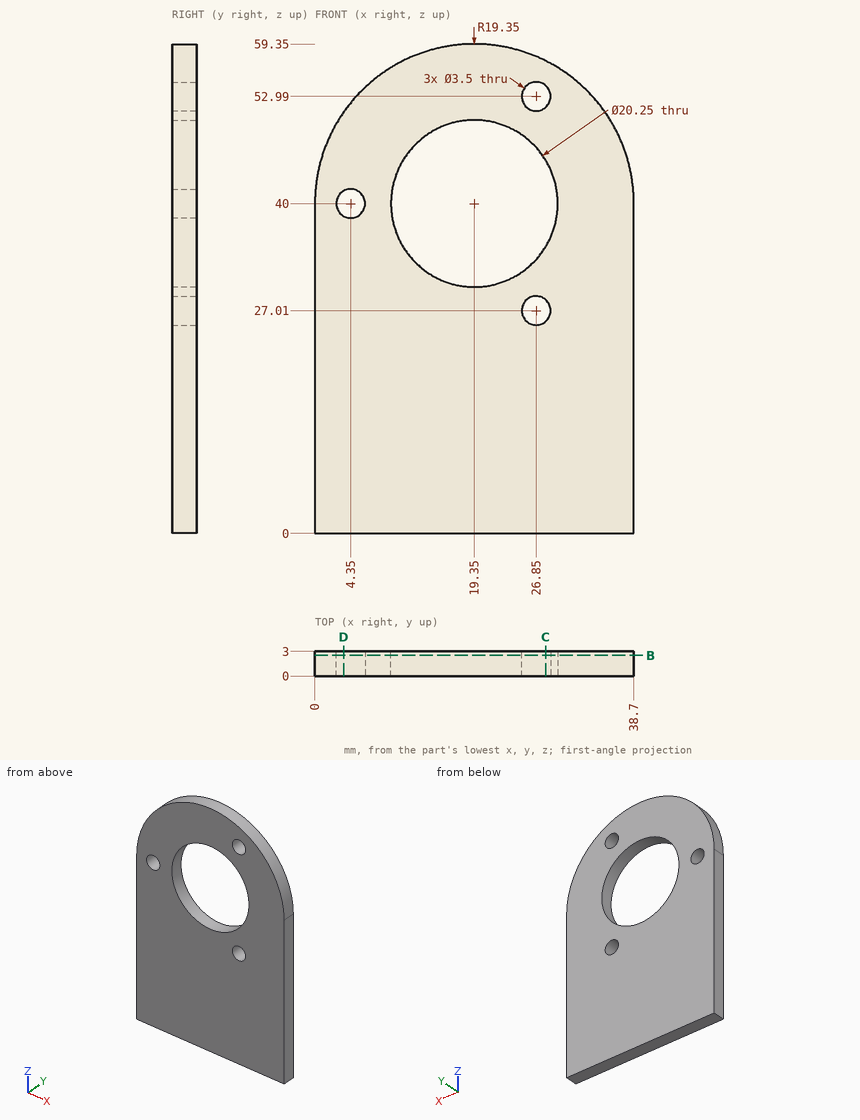
Drawing for the job (mm, zero at the part's lowest x, y, z). Give positions to 0.01 mm unless a question says otherwise; leave off trailing zeros. Order: outer loops, then holes, each group sorted by start corner. A loop starts at its lowest first (then second) coordinate and runs counter-clockwise, first axis right, second up. Notation, with made-up numbers: (-4, 73.25) -> (8, 73.25) arc R21 cw to (8, 110.25) -> close; hole circle Ø8 at (31, 51.25). An arc over 180 degrees is marked (long way). Use one line per item in the form item = value.
(1) Saw through at C-C (x = 28). Write the cut outline in (y, z).
Solution:
outline = (0, 0) -> (3, 0) -> (3, 25.69) -> (0, 25.69) -> close; (0, 28.33) -> (3, 28.33) -> (3, 34.74) -> (0, 34.74) -> close; (0, 45.26) -> (3, 45.26) -> (3, 51.67) -> (0, 51.67) -> close; (0, 54.31) -> (3, 54.31) -> (3, 57.31) -> (0, 57.31) -> close
(2) Drill centre lines: line 1 (Z direction, x = 27, y = 1.95) (1 decimal); line 2 (Z direction, x = 11, y = 2.7) (1 decimal); line 3 (X direction, y = 1, z = 32.5). Where is each one in solid material? Low to high. Write a range as from..to.
Solution:
line_1 = 0..25.3, 28.8..33.4, 46.6..51.2, 54.7..57.8
line_2 = 0..34.3, 45.7..57.5
line_3 = 0..12.55, 26.15..38.7
(3) Saw through at B-B (y = 2.5). Count the separate pieces of the cut face and the enclosed holes in it, then the cut area to 4 significant figures.
Solution:
separate_pieces = 1
enclosed_holes = 4
area = 1,785 mm²
(4) Saw through at D-D (x = 3.5). Write the cut outline in (y, z), then the cut area to 3 significant figures.
Solution:
outline = (0, 0) -> (3, 0) -> (3, 38.47) -> (0, 38.47) -> close; (0, 41.53) -> (3, 41.53) -> (3, 51.1) -> (0, 51.1) -> close
area = 144 mm²
(5) Flat gauge pin, fed straight in: P1, Ø1, axis at x = 9, y = 1.5, coming from the +Z side (1 decimal). Where does the tip first touch, or does it go through?
Solution:
P1 = 56.7
